from build123d import *

# Parameters (mm, degrees)
BOSS_EXTRUDE1_DEPTH      = 4
BOSS_EXTRUDE1_DEPTH_BACK = 4
BOSS_EXTRUDE2_START      = 4
SKETCH1_3_R              = 5
BOSS_EXTRUDE2_DEPTH      = 9
SKETCH2_R                = 1.5
CUT_EXTRUDE1_DEPTH       = 17
SKETCH3_R                = 18.5
BOSS_EXTRUDE3_DEPTH      = 6
SKETCH4_R                = 8
SKETCH4_R_2              = 1.5
CUT_EXTRUDE2_DEPTH       = 14
FILLET1_R                = 10


with BuildPart() as part:
    # Sketch1 → Boss-Extrude1 (new, two sides: drawn at the far end of the back side and taken through both)
    with BuildSketch(Plane(origin=(0, 0, 0), x_dir=(0, 0, -1), z_dir=(1, 0, 0)).offset(-BOSS_EXTRUDE1_DEPTH_BACK)):
        with BuildLine():
            Line((-7, -14.38749457), (-7, -29.38749457))
            ThreePointArc((-7, -29.38749457), (-16, -43.77498914), (-7, -58.16248371))
            Line((-7, -58.16248371), (-7, -88.16248371))
            ThreePointArc((-7, -88.16248371), (0, -129.99103506), (7, -88.16248371))
            Line((7, -88.16248371), (7, -58.16248371))
            ThreePointArc((7, -58.16248371), (16, -43.77498914), (7, -29.38749457))
            Line((7, -29.38749457), (7, -14.38749457))
            ThreePointArc((7, -14.38749457), (0, 16), (-7, -14.38749457))
        make_face()
    extrude(amount=BOSS_EXTRUDE1_DEPTH + BOSS_EXTRUDE1_DEPTH_BACK)

    # Sketch1<3> → Boss-Extrude2 (add)
    with BuildSketch(Plane(origin=(0, 0, 0), x_dir=(0, 0, -1), z_dir=(1, 0, 0)).offset(BOSS_EXTRUDE2_START)):
        Circle(SKETCH1_3_R)
        with Locations((0, -43.77498914)):
            Circle(SKETCH1_3_R)
    extrude(amount=BOSS_EXTRUDE2_DEPTH)

    # Sketch2 → Cut-Extrude1 (cut)
    with BuildSketch(Plane.ZY.offset(4)):
        Circle(SKETCH2_R)
        with Locations((0, -43.77498914)):
            Circle(SKETCH2_R)
    extrude(amount=-CUT_EXTRUDE1_DEPTH, mode=Mode.SUBTRACT)

    # Sketch3 → Boss-Extrude3 (add)
    with BuildSketch(Plane(origin=(4, 0, 0), x_dir=(0, 0, -1), z_dir=(1, 0, 0))):
        with BuildLine():
            ThreePointArc((-7, -88.16248371), (-12.484990989, -125.994606124), (21.5, -108.49103506))
            ThreePointArc((21.5, -108.49103506), (17.503571064, -96.006044071), (7, -88.16248371))
            ThreePointArc((7, -88.16248371), (0, -86.99103506), (-7, -88.16248371))
        make_face()
        with Locations((0, -108.49103506)):
            Circle(SKETCH3_R, mode=Mode.SUBTRACT)
    extrude(amount=BOSS_EXTRUDE3_DEPTH)

    # Sketch4 → Cut-Extrude2 (cut)
    with BuildSketch(Plane.ZY.offset(4)):
        with Locations((0, -115.49103506)):
            Circle(SKETCH4_R)
        with Locations((15.496292799, -108.49103506)):
            Circle(SKETCH4_R_2)
        with Locations((7.7481464, -95.070851831)):
            Circle(SKETCH4_R_2)
        with Locations((-7.7481464, -95.070851831)):
            Circle(SKETCH4_R_2)
        with Locations((-15.496292799, -108.49103506)):
            Circle(SKETCH4_R_2)
        with Locations((-7.7481464, -121.911218289)):
            Circle(SKETCH4_R_2)
        with Locations((7.7481464, -121.911218289)):
            Circle(SKETCH4_R_2)
    extrude(amount=-CUT_EXTRUDE2_DEPTH, mode=Mode.SUBTRACT)

    # Fillet1
    # the kernel refuses this fillet: 10 mm, written as the material it adds along each edge
    with BuildSketch(Plane(origin=(-4, -29.38749457, 7), x_dir=(0, 1, 0), z_dir=(1, 0, 0)), Plane(origin=(4, -14.38749457, 7), x_dir=(0, -1, 0), z_dir=(-1, 0, 0)), Plane(origin=(4, -29.38749457, -7), x_dir=(0, 1, 0), z_dir=(-1, 0, 0))) as fillet1_piece_1:
        with BuildLine():
            CenterArc((5.284821003, 10), FILLET1_R, 220.832217027, 49.167782973)
            ThreePointArc((-2.281454217, 3.461538462), (-1.028137912, 1.804975281), (0, 0))
            Line((0, 0), (5.284821003, 0))
        make_face()
    extrude(amount=8)
    with BuildSketch(Plane(origin=(4, -14.38749457, -7), x_dir=(0, 0.5503109550569161, -0.8349597910943646), z_dir=(-1, 0, 0)), Plane(origin=(-4, -58.16248371, 7), x_dir=(0, 0.5503109550569153, 0.8349597910943651), z_dir=(1, 0, 0))) as fillet1_piece_2:
        with BuildLine():
            CenterArc((5.441303017, 9.915722591), FILLET1_R, 213.3883484, 49.167782973)
            Line((-2.908294893, 4.412613041), (0, 0))
            ThreePointArc((0, 0), (2.07287734, 0.134843854), (4.14575468, 0))
        make_face()
    extrude(amount=8)
    with BuildSketch(Plane(origin=(-4, -58.16248371, -7), x_dir=(0, 0.5503109550569155, -0.834959791094365), z_dir=(1, 0, 0))) as fillet1_piece_3:
        with BuildLine():
            CenterArc((5.441303017, -9.915722591), FILLET1_R, 97.443868628, 49.167782973)
            Line((-2.908294893, -4.412613041), (0, 0))
            ThreePointArc((0, 0), (2.07287734, -0.134843854), (4.14575468, 0))
        make_face()
    extrude(amount=8)
    with BuildSketch(Plane(origin=(-4, -88.16248371, -7), x_dir=(0, 1, 0), z_dir=(1, 0, 0))) as fillet1_piece_4:
        with BuildLine():
            CenterArc((6.190309862, -10), FILLET1_R, 90, 57.337969437)
            ThreePointArc((-2.228376237, -4.603174603), (-0.976831569, -2.368080993), (0, 0))
            Line((0, 0), (6.190309862, 0))
        make_face()
    extrude(amount=8)
    with BuildSketch(Plane(origin=(-4, -88.16248371, 7), x_dir=(0, -0.43572469735161884, 0.9000799898441472), z_dir=(1, 0, 0))) as fillet1_piece_5:
        with BuildLine():
            CenterArc((6.303529007, -9.929021011), FILLET1_R, 96.8306141, 57.337969437)
            Line((-2.697270891, -5.571774038), (0, 0))
            ThreePointArc((0, 0), (2.557091956, -0.152604826), (5.114183912, 0))
        make_face()
    extrude(amount=8)


solid = part.part
Verification items for the finished model (mm, model axes). A direction names the side the tool comes from. Give positions to 0.01 mm unless a question says otherwise; leave off trailing zeros. Order: outer loops, then holes, each group sorted by start corner. A loop starts at its lowest first (then second) coordinate and runs counter-clockwise, first axis right, second up. Notation, with made-up numbers: (81.5, 77.25) -> (137.5, 77.25) arc R8 cw to (137.5, 86.25) -> close; hole circle Ø11 at (27.5, 39.5). An arc over 180 degrees is marked (long way). Answer as CSV lines item,"result".
Q1. Depth check by flat-ended pin: pin 1 (6.5 mm diameter, centred on x = 0.5, y = -71, fed in from +Z); pin 2 (8 mm diameter, centred on x = 6, z = -6.5, fed in from -Y); pin 3 (1.5 mm diameter, centred on x = 9, y = -100.5, fed in from +Z); pin 4 (2.5 mm diameter, centred on y = -121.91, z = -7.75, fed in from +X). Enter the tip coordinate at first touch or a pass-through.
Solutions:
pin 1,"stops at z = 7"
pin 2,"stops at y = -129.85"
pin 3,"stops at z = 20.24"
pin 4,"passes through"
Q2. Access from +Z, -Z, +X, -X, +Y, -Y to the whole of each face (thin tool, end or side, straight path). Record for faces 1 (the flat face through (10, -92, -9)), 2 (the cylindrical face through (-0.056, -86.708, -8.193)), 3 (the cylindrical face through (-0.056, -28.317, 7.932)).
Solutions:
face 1,"+Z, -Z, +X, -Y"
face 2,"-Z, +X, -X"
face 3,"+Z, +X, -X"
Q3. Scan lines: probe 1 along Y at (x, z) = (-0.75, 0); probe 2 along Y at (x, z) = (-1, 0.5); probe 3 along X at (y, z) = (-30, 6). Record each from-to range of solid material in increasing order.
Solutions:
probe 1,"y = -129.99 to -123.49, -107.49 to -45.27, -42.27 to -1.5, 1.5 to 16"
probe 2,"y = -129.99 to -123.48, -107.51 to -45.19, -42.36 to -1.41, 1.41 to 15.99"
probe 3,"x = -4 to 4"
Q4. Release check for a two-part mould opening along Z. For faces 4 (the cylindrical face through (0, -44, 16)), 5 (the cylindrical face through (0.06, -15.57, -7.88)), 6 (the flat face through (4, -104, 0)) record: +Z half, -Z half, draft (parallel to the pull), parting line (faces both ways), or undercut.
Solutions:
face 4,"+Z half"
face 5,"-Z half"
face 6,"undercut"
Q5. Sectioned sample at D-D on y = -53. Record the cut outline in (x, z), plus the area to 3 significant figures.
Solutions:
outline,"(-4, -13.07) -> (4, -13.07) -> (4, 13.07) -> (-4, 13.07) -> close"
area,"209 mm²"
Q6. Sectioned sample at C-C on x = 8.5. Record the cut outline in (y, z), plus the area to 3 significant figures.
Solutions:
outline,"circle Ø43 at (-108.49, 0); circle Ø10 at (-43.77, 0); circle Ø10 at (0, 0); hole circle Ø37 at (-108.49, 0); hole circle Ø3 at (-43.77, 0); hole circle Ø3 at (0, 0)"
area,"520 mm²"
Q7. Sectioned sample at B-B on y = 0. Record the cut outline in (x, z), plus the area to 3 significant figures.
Solutions:
outline,"(-4, -16) -> (4, -16) -> (4, -5) -> (13, -5) -> (13, -1.5) -> (-4, -1.5) -> close; (-4, 1.5) -> (13, 1.5) -> (13, 5) -> (4, 5) -> (4, 16) -> (-4, 16) -> close"
area,"295 mm²"
Q8. Sectioned sample at A-A on z = 0. Count the separate pieces of the cut face and the enclosed holes in it, plus the area to 3 significant figures.
Solutions:
separate pieces,"4"
enclosed holes,"0"
area,"1,150 mm²"
